```python
from build123d import *

# Parameters (mm, degrees)
F0_R     = 17.5
F0_R_2   = 4
F1_DEPTH = 3
F2_DEPTH = 55
F3_R     = 10
F3_R_2   = 4
F4_DEPTH = 3


with BuildPart() as f1:
    # F0 (on Top) → F1 (new body)
    with BuildSketch(Plane.XY):
        Circle(F0_R)
        Circle(F0_R_2, mode=Mode.SUBTRACT)
        Circle(F0_R_2)
    extrude(amount=F1_DEPTH)

    # F0 (on Top) → F2 (join)
    with BuildSketch(Plane.XY):
        Circle(F0_R_2)
    extrude(amount=F2_DEPTH)

    # F3 (on face) → F4 (join)
    with BuildSketch(Plane.XY.offset(55)):
        Circle(F3_R)
        Circle(F3_R_2)
    extrude(amount=F4_DEPTH)


solid = f1.part
```
The listing builds one solid part. Answer for the finished solid, in the listing's coordinates (mm). A direction names the side the tool comes from. Coordinates: 2 decimals unless noted, no trailing zeros. Write each loop counter-clockwise with the first axis right and the second up, starting at its lowest first coordinate (ties: lowest second). Pieces come first, ordered by that corner, then holes. Notation, with made-up numbers: (-21, 54) -> (26, 54) arc R12 ccw to (26, 73) -> close; hole circle Ø9 at (-25.75, 16.5). An arc over 180 degrees is marked (long way). Write each question's results on one line, items separated by ' | '. Start each with the question number.
1) A tool of negligible diameter and unlimited length cuts with its end or side. For faces 1 (the cylindrical face through (-13.887, -10.648, 1.479)), 2 (the cylindrical face through (-2.17, -9.76, 56.48)), 3 (the cylindrical face through (-0.867, -3.905, 28.636)), from which of +Z, -Z, +X, -X, +Y, -Y can it reach the whole face along a straight path? Write none if from no direction.
2) Straight lines are drawn through the part: probe 1 along Z at (x, y) = (-3.5, -9); probe 2 along Z at (x, y) = (3.5, 14.5); probe 3 along X at (y, z) = (0, 15.5). For each, find the intervals that lie inside material, in ascending order.
3) Flat-ended cylindrical pins translate along their axes: pin 1 Ø16 at (x, y) = (-1, 1) entering from -Z; pin 2 Ø1 at (x, y) = (9.5, 13.5) entering from +Z; pin 3 Ø8 at (x, z) = (-9.5, 29.5) entering from +Y; pin 4 Ø1 at (y, z) = (-3.5, 33.5) entering from -X. Find the tip coordinate at first contact, or state that the pin passes through.
4) For a pull along Z with two mould halves and no side action, classify faces 4 (the flat face through (0, 0, 58)), 5 (the flat face through (4, -4, 3)), 6 (the flat face through (0, 0, 0)) as +Z half, -Z half, draft (parallel to the pull), parting line (faces both ways), or undercut.
5) A cutting plane is placed at A-A (x = 0). Determine the outline of the cut face in (y, z).
6) A cutting plane is placed at B-B (x = 7). Determine the outline of the cut face in (y, z).
7) A cutting plane is placed at D-D (z = 51). Determine the outline of the cut face in (x, y).
Values follow:
1) face 1: +Z, -Z | face 2: +Z | face 3: none
2) probe 1: 0 to 3, 55 to 58 | probe 2: 0 to 3 | probe 3: -4 to 4
3) pin 1: z = 0 | pin 2: z = 3 | pin 3: through | pin 4: x = -2.65
4) face 4: +Z half | face 5: undercut | face 6: -Z half
5) outline: (-17.5, 0) -> (17.5, 0) -> (17.5, 3) -> (4, 3) -> (4, 55) -> (10, 55) -> (10, 58) -> (-10, 58) -> (-10, 55) -> (-4, 55) -> (-4, 3) -> (-17.5, 3) -> close
6) outline: (-16.04, 0) -> (16.04, 0) -> (16.04, 3) -> (-16.04, 3) -> close; (-7.14, 55) -> (7.14, 55) -> (7.14, 58) -> (-7.14, 58) -> close
7) outline: circle Ø8 at (0, 0)
